Build history of the part. All positions in model axes, mm. Face numbers are marked on the shaded views. Give positions to 0.01 mm unless a question says otherwise; leave off trailing zeros. Write each loop counter-clockwise with the first axis right and the second up, starting at its lowest first coordinate (ties: lowest second). Pieces come first, ordered by that corner, then holes. Notation, with made-up numbers: M -34,-40 L 7,-40 A15 ccw 7,-24 Z; hole C 40.5,28 d5. An arc over 180 degrees is marked long. One line per item, written item: value. Start each with the question number.
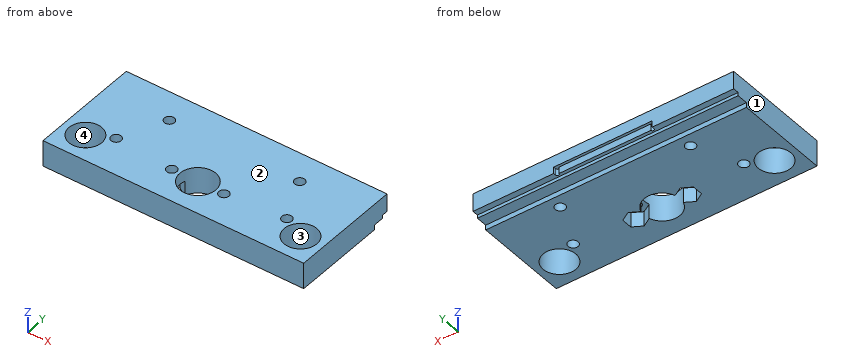
from build123d import *

# Parameters (mm, degrees)
SKETCH_2_W           = 80
SKETCH_2_H           = 34
SKETCH_2_R           = 5.025
SKETCH_2_R_2         = 4.05
EXTRUDE_1_DEPTH      = 8
CUT_EXTRUDE_2_DEPTH  = 88.292611371
SKETCH_5_R           = 1.55
CUT_EXTRUDE_3_DEPTH  = 88.292611371
CUT_EXTRUDE_5_DEPTH  = 4.5
SKETCH_11_R          = 1.55
CUT_EXTRUDE_7_DEPTH  = 88.292611371
CUT_EXTRUDE_11_DEPTH = 2
SKETCH_22_R          = 1.55
CUT_EXTRUDE_13_DEPTH = 88.292611371
SKETCH_20_R          = 5.5
CUT_EXTRUDE_14_DEPTH = 88.292611371


with BuildPart() as part:
    # 草图2 → 凸台-拉伸1 (new body)
    with BuildSketch(Plane.XY):
        with Locations((40, 17)):
            Rectangle(SKETCH_2_W, SKETCH_2_H)
        with Locations((7, 8)):
            Circle(SKETCH_2_R, mode=Mode.SUBTRACT)
        with Locations((40, 10)):
            Circle(SKETCH_2_R_2, mode=Mode.SUBTRACT)
        with Locations((73, 8)):
            Circle(SKETCH_2_R, mode=Mode.SUBTRACT)
    extrude(amount=EXTRUDE_1_DEPTH)

    # 草图4 → 切除-拉伸2 (cut, through all)
    with BuildSketch(Plane(origin=(80, 0, 0), x_dir=(0, 0, -1), z_dir=(1, 0, 0))):
        Polygon((-1.5, 32.2), (-2.5, 32.2), (-2.5, 34), (0, 34), (0, 28.8), (-1.5, 28.8), align=None)
    extrude(amount=-CUT_EXTRUDE_2_DEPTH, mode=Mode.SUBTRACT)

    # 草图5 → 切除-拉伸3 (cut, through all)
    with BuildSketch(Plane.XY.offset(8)):
        with Locations((48, 10)):
            Circle(SKETCH_5_R)
        with Locations((32, 10)):
            Circle(SKETCH_5_R)
    extrude(amount=-CUT_EXTRUDE_3_DEPTH, mode=Mode.SUBTRACT)

    # 草图8 → 切除-拉伸5 (cut)
    with BuildSketch(Plane(origin=(0, 0, 0), x_dir=(-1, 0, 0), z_dir=(0, 0, -1))):
        Polygon((-45.15, 8.354551733), (-45.15, 11.645448267), (-48, 13.290896534), (-50.85, 11.645448267), (-50.85, 8.354551733), (-48, 6.709103466), align=None)
        Polygon((-34.85, 8.354551733), (-32, 6.709103466), (-29.15, 8.354551733), (-29.15, 11.645448267), (-32, 13.290896534), (-34.85, 11.645448267), align=None)
    extrude(amount=-CUT_EXTRUDE_5_DEPTH, mode=Mode.SUBTRACT)

    # 草图11 → 切除-拉伸7 (cut, through all)
    with BuildSketch(Plane(origin=(0, 0, 0), x_dir=(-1, 0, 0), z_dir=(0, 0, -1))):
        with Locations((-60, 25)):
            Circle(SKETCH_11_R)
        with Locations((-20, 25)):
            Circle(SKETCH_11_R)
    extrude(amount=-CUT_EXTRUDE_7_DEPTH, mode=Mode.SUBTRACT)

    # 草图19 → 切除-拉伸11 (cut)
    with BuildSketch(Plane(origin=(0, 0, 2.5), x_dir=(-1, 0, 0), z_dir=(0, 0, -1))):
        with BuildLine():
            Line((-25, 34), (-55.247938178, 34))
            Line((-55.247938178, 34), (-55.247938178, 33.2))
            ThreePointArc((-55.247938178, 33.2), (-54.747938178, 32.7), (-54.247938178, 33.2))
            Line((-54.247938178, 33.2), (-26, 33.2))
            ThreePointArc((-26, 33.2), (-25.5, 32.7), (-25, 33.2))
            Line((-25, 33.2), (-25, 34))
        make_face()
    extrude(amount=-CUT_EXTRUDE_11_DEPTH, mode=Mode.SUBTRACT)

    # 草图22 → 切除-拉伸13 (cut, through all)
    with BuildSketch(Plane(origin=(0, 0, 0), x_dir=(-1, 0, 0), z_dir=(0, 0, -1))):
        with Locations((-66.2, 11.5)):
            Circle(SKETCH_22_R)
        with Locations(Location((-13.8, 11.5, 0), (0, 0, 180))):
            Circle(SKETCH_22_R)
    extrude(amount=-CUT_EXTRUDE_13_DEPTH, mode=Mode.SUBTRACT)

    # 草图20 → 切除-拉伸14 (cut, through all)
    with BuildSketch(Plane(origin=(0, 0, 0), x_dir=(-1, 0, 0), z_dir=(0, 0, -1))):
        with Locations((-40, 10)):
            Circle(SKETCH_20_R)
    extrude(amount=-CUT_EXTRUDE_14_DEPTH, mode=Mode.SUBTRACT)


solid = part.part
1) Band-saw the part on D-D (x = 40). List the corners of the cut face in (y, z), then the cut area to 3 significant figures.
2) Probe line 1 along Y through (x, z) = (66.2, 4.25); line 2 along Y through (x, z) = (73, 5.25) (3 decimals); line 3 along X through (y, z) = (8.5, 0.5). List the from-to ranges inside material, lowest first. Write a range as from..to.
3) Drop flat-ended pins along their axis: P1, Ø0.9, axis at y = 33.5, z = 3.5, coming from the -X side; P2, Ø1.9, axis at x = 66.2, y = 11.5, coming from the +Z side; P3, Ø1.2, axis at x = 28.5, z = 1, coming from the +Y side; P4, Ø0.6, axis at x = 46, y = 33, coming from the -Z side. Give the stop position or say it passes through.
4) Band-saw the part on C-C (y = 25). List the corners of the cut face in (x, z).
5) Band-saw the part on B-B (z = 5.25). Count the separate pieces of the cut face and the enclosed holes in it, then the cut area to 3 significant figures.
6) Mould opens along X. For the marked faces 1, 2, 3 and 4 say: released by +X, released by -X, zero draft, split by the parting line, or undercut.
7) Band-saw the part on A-A (x = 20). List the corners of the cut face in (y, z).
Model answer:
1. outline: M 0,0 L 4.5,0 L 4.5,8 L 0,8 Z; M 15.5,0 L 28.8,0 L 28.8,1.5 L 32.2,1.5 L 32.2,2.5 L 33.2,2.5 L 33.2,4.5 L 34,4.5 L 34,8 L 15.5,8 Z
1. area: 173 mm²
2. line 1: y = 0..9.95, 13.05..34
2. line 2: y = 0..2.975, 13.025..34
2. line 3: x = 0..2, 12..29.15, 50.85..68, 78..80
3. P1: stops at x = 0
3. P2: passes through
3. P3: stops at y = 32.2
3. P4: stops at z = 2.5
4. outline: M 0,0 L 18.45,0 L 18.45,8 L 0,8 Z; M 21.55,0 L 58.45,0 L 58.45,8 L 21.55,8 Z; M 61.55,0 L 80,0 L 80,8 L 61.55,8 Z
5. separate pieces: 1
5. enclosed holes: 9
5. area: 2,420 mm²
6. face 1: released by -X
6. face 2: zero draft
6. face 3: undercut
6. face 4: undercut
7. outline: M 0,0 L 23.45,0 L 23.45,8 L 0,8 Z; M 26.55,0 L 28.8,0 L 28.8,1.5 L 32.2,1.5 L 32.2,2.5 L 34,2.5 L 34,8 L 26.55,8 Z
